Design review of the part built by this model. Coordinates are the model's own, in mm. Face numbers are marked on the shaded views. A direction names the side the tool comes from. Coordinates: 2 decimals unless noted, no trailing zeros. Loops run counter-clockwise (first coordinate to the right, second up) from the corner with the lowest first, then second, coordinate; pieces in that order, holes last. Notation, with made-up numbers: (73.5, 59.25) - (83.5, 59.25) arc R24 cw to (83.5, 81.25) - close; hole circle Ø4 at (47, -14). An arc over 180 degrees is marked (long way). Return JSON: item names as keys, results as strings. Group by question number.
from build123d import *

# Parameters (mm, degrees)
SKETCH1_R           = 10
BOSS_EXTRUDE1_DEPTH = 48
BOSS_EXTRUDE3_START = 2
SKETCH3_R           = 12.5
SKETCH3_R_2         = 3.5
SKETCH3_R_3         = 0.95
BOSS_EXTRUDE3_DEPTH = 2
SKETCH4_R           = 2.38125
CUT_EXTRUDE1_DEPTH  = 61.153219082
SKETCH6_W           = 58.309477214
SKETCH6_H           = 41.572471276
SKETCH6_R           = 12.5
CUT_EXTRUDE4_DEPTH  = 22


with BuildPart() as part:
    # Sketch1 → Boss-Extrude1 (new body)
    with BuildSketch(Plane.XY):
        with BuildLine():
            Line((-25, 13.756613757), (-25, 11.243386243))
            Line((-25, 11.243386243), (-22.480898871, 11.243386243))
            ThreePointArc((-22.480898871, 11.243386243), (-15.409831059, 8.314454055), (-12.480898871, 1.243386243))
            Line((-12.480898871, 1.243386243), (-12.480898871, 0.690770135))
            ThreePointArc((-12.480898871, 0.690770135), (0, -12.5), (12.480898871, 0.690770135))
            Line((12.480898871, 0.690770135), (12.480898871, 1.243386243))
            ThreePointArc((12.480898871, 1.243386243), (15.409831059, 8.314454055), (22.480898871, 11.243386243))
            Line((22.480898871, 11.243386243), (25, 11.243386243))
            Line((25, 11.243386243), (25, 13.756613757))
            Line((25, 13.756613757), (-25, 13.756613757))
        make_face()
        Circle(SKETCH1_R, mode=Mode.SUBTRACT)
    extrude(amount=BOSS_EXTRUDE1_DEPTH)

    # Sketch3 → Boss-Extrude3 (add)
    with BuildSketch(Plane(origin=(0, 0, 0), x_dir=(-1, 0, 0), z_dir=(0, 0, -1)).offset(BOSS_EXTRUDE3_START)):
        Circle(SKETCH3_R)
        Circle(SKETCH3_R_2, mode=Mode.SUBTRACT)
        with Locations((7.5, 0)):
            Circle(SKETCH3_R_3, mode=Mode.SUBTRACT)
        with Locations((-7.5, 0)):
            Circle(SKETCH3_R_3, mode=Mode.SUBTRACT)
    extrude(amount=-BOSS_EXTRUDE3_DEPTH)

    # Sketch4 → Cut-Extrude1 (cut, through all)
    with BuildSketch(Plane(origin=(0, 13.756613757, 0), x_dir=(1, 0, 0), z_dir=(0, 1, 0))):
        with Locations(Location((-20, -25, 0), (0, 0, 270))):
            Circle(SKETCH4_R)
        with Locations(Location((20, -25, 0), (0, 0, 270))):
            Circle(SKETCH4_R)
        with Locations(Location((20, -43, 0), (0, 0, 270))):
            Circle(SKETCH4_R)
        with Locations(Location((-20, -43, 0), (0, 0, 270))):
            Circle(SKETCH4_R)
    extrude(amount=-CUT_EXTRUDE1_DEPTH, mode=Mode.SUBTRACT)

    # Sketch6 → Cut-Extrude4 (cut)
    with BuildSketch(Plane(origin=(0, 0, -2), x_dir=(-1, 0, 0), z_dir=(0, 0, -1))):
        Rectangle(SKETCH6_W, SKETCH6_H)
        Circle(SKETCH6_R, mode=Mode.SUBTRACT)
    extrude(amount=-CUT_EXTRUDE4_DEPTH, mode=Mode.SUBTRACT)


solid = part.part
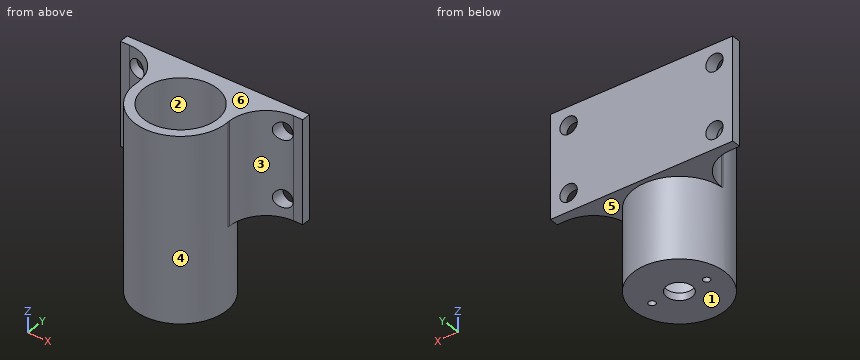
Item 1: Add section D-D (y = 0). State the section outline as (x, z) points, then the cut area to 3 significant figures.
Item 2: Add section C-C (z = 44). State the section outline as (x, y) points.
Item 3: Add section B-B (z = 29.5). State the section outline as (x, y) points, then the cut area to 3 significant figures.
Item 4: Draft analysis for pull direction X (two halves, no side actions). For the marked faces 1, 2 and 3, state which applies: pulls with the +X half, pulls with the -X half, needs draft (parallel to the pull), parting line crosses it, or undercut.
Item 5: For P1, Ø10, axis at y = 9, z = 11, coming from the +X side; P2, Ø2, axis at x = 10, z = 23.5, coming from the -Y side; P3, Ø2, axis at x = -23.5, z = 38, coming from the -Y side, all flat-tipped, find the tip position at first contact; note any pin that passes through.
Item 6: Add section A-A (x = 0). State the section outline as (y, z) points, then the cut area to 3 significant figures.
Item 7: For the marked faces 4, 5 and 6, list the 3-axis set-ups (+Z, -Z, +X, -X, +Y, -Y) from which the entire face can be reached by the end or side of a thin tool; tool diameter is ignored.
Item 8: To check wall thickness, follow line 1 (X direction, y = 11.75, z = 43); line 2 (Z direction, x = 20, y = 11.9); line 3 (Y direction, x = 7.5, z = -1.1). State the ranges of each line that lie inside material, in increasing order. Write a range as from..to.
Answers below:
{
 "1": {"outline": "(-12.5, -2) - (-8.45, -2) - (-8.45, 0) - (-10, 0) - (-10, 48) - (-12.5, 48) - close; (-6.55, -2) - (-3.5, -2) - (-3.5, 0) - (-6.55, 0) - close; (3.5, -2) - (6.55, -2) - (6.55, 0) - (3.5, 0) - close; (8.45, -2) - (12.5, -2) - (12.5, 48) - (10, 48) - (10, 0) - (8.45, 0) - close", "area": "268 mm^2"},
 "2": {"outline": "(-25, 11.24) - (-22.48, 11.24) arc R10 cw to (-22.16, 11.24) - (-22.16, 13.76) - (-25, 13.76) - close; (-17.84, 10.1) arc R10 cw to (-12.48, 1.24) - (-12.48, 0.69) arc R12.5 ccw (long way) to (12.48, 0.69) - (12.48, 1.24) arc R10 cw to (17.84, 10.1) - (17.84, 13.76) - (-17.84, 13.76) - close; (22.16, 11.24) arc R10 cw to (22.48, 11.24) - (25, 11.24) - (25, 13.76) - (22.16, 13.76) - close; hole circle Ø20 at (0, 0)"},
 "3": {"outline": "(-25, 11.24) - (-22.48, 11.24) arc R10 cw to (-12.48, 1.24) - (-12.48, 0.69) arc R12.5 ccw (long way) to (12.48, 0.69) - (12.48, 1.24) arc R10 cw to (22.48, 11.24) - (25, 11.24) - (25, 13.76) - (-25, 13.76) - close; hole circle Ø20 at (0, 0)", "area": "381 mm^2"},
 "4": {"face 1": "needs draft", "face 2": "undercut", "face 3": "pulls with the +X half"},
 "5": {"P1": "stops at x = 11.84", "P2": "stops at y = -8.67", "P3": "stops at y = 11.24"},
 "6": {"outline": "(-12.5, -2) - (-3.5, -2) - (-3.5, 0) - (-10, 0) - (-10, 48) - (-12.5, 48) - close; (3.5, -2) - (12.5, -2) - (12.5, 20) - (13.76, 20) - (13.76, 48) - (10, 48) - (10, 0) - (3.5, 0) - close", "area": "311 mm^2"},
 "7": {"face 4": "-Z", "face 5": "-Z, +Y", "face 6": "+Z, +X, -X, +Y, -Y"},
 "8": {"line 1": "x = -25..-22.38, -17.62..17.62, 22.38..25", "line 2": "z = 20..22.62, 27.38..40.62, 45.38..48", "line 3": "y = -10..-0.95, 0.95..10"}
}
